Geometry: final body of the model. Coordinates: model frame, mm. A direction names the side the tool comes from. Give positions to 0.01 mm unless a question says otherwise; leave off trailing zeros. Loops run counter-clockwise (first coordinate to the right, second up) from the corner with the lowest first, then second, coordinate; pieces in that order, holes last. Notation, with made-up numbers: (63.25, 43.25) - (86.25, 43.25) arc R19 ccw to (86.25, 66.25) - close; hole circle Ø8 at (-3, 36). An arc over 180 degrees is marked (long way). Use one line per item in the form item = value.
```python
from build123d import *

# Parameters (mm, degrees)
SKETCH1_R    = 5
SPIGOT_DEPTH = 14
BODY_START   = 14
SKETCH2_R    = 7
BODY_DEPTH   = 22
SPOUT_START  = -38
SKETCH3_R    = 5
SPOUT_DEPTH  = 38
LEVER_START  = 6
SKETCH4_W    = 10
SKETCH4_H    = 6
LEVER_DEPTH  = 22


with BuildPart() as part:
    # Sketch1 → Spigot (new body)
    with BuildSketch(Plane.XY):
        Circle(SKETCH1_R)
    extrude(amount=SPIGOT_DEPTH)

    # Sketch2 → Body (add)
    with BuildSketch(Plane.XY.offset(BODY_START)):
        Circle(SKETCH2_R)
    extrude(amount=BODY_DEPTH)

    # Sketch3 → Spout (add)
    with BuildSketch(Plane(origin=(0, 0, 0), x_dir=(1, 0, 0), z_dir=(0, 1, 0)).offset(SPOUT_START)):
        with Locations(Location((0, -30, 0), (0, 0, 90))):
            Circle(SKETCH3_R)
    extrude(amount=SPOUT_DEPTH)

    # Sketch4 → Lever (add)
    with BuildSketch(Plane(origin=(0, 0, 0), x_dir=(1, 0, 0), z_dir=(0, 1, 0)).offset(LEVER_START)):
        with Locations((0, -26)):
            Rectangle(SKETCH4_W, SKETCH4_H)
    extrude(amount=LEVER_DEPTH)


solid = part.part
```
(1) Access query for faces 1 (the face through (-1.5, -21.68, 25.23)), 2 (the face through (-1.08, -4.88, 6.9)), 3 (the face through (-5, 17, 26)), 4 (the face through (5, 17, 26)). Directions: +Z, -Z, +X, -X, +Y, -Y. A direction counts if a zero-diameter tool reaches every point of the face in a straight line with its end or side. Return the directions, or none.
Solution:
face_1 = -Y
face_2 = -Z
face_3 = +Z, -Z, -X, +Y
face_4 = +Z, -Z, +X, +Y
(2) Cut plane B-B (y = 0). Return the cut outline in (x, z).
Solution:
outline = (-7, 14) - (-5, 14) - (-5, 0) - (5, 0) - (5, 14) - (7, 14) - (7, 36) - (-7, 36) - close
(3) Material intervals for L1, parallel to Y at x = 0, z = 19; L2, parallel to Z at x = -1.25, y = 23; L3, parallel to Z at x = 6.25, y = -2.5, sorted ascending. Write a range as from..to.
Solution:
L1 = -7..7
L2 = 23..29
L3 = 14..36
(4) Cut plane D-D (x = 2.75). Return the cut outline in (y, z), plus the area to 3 significant figures.
Solution:
outline = (-38, 25.82) - (-6.44, 25.82) - (-6.44, 14) - (-4.18, 14) - (-4.18, 0) - (4.18, 0) - (4.18, 14) - (6.44, 14) - (6.44, 23) - (28, 23) - (28, 29) - (6.44, 29) - (6.44, 36) - (-6.44, 36) - (-6.44, 34.18) - (-38, 34.18) - close
area = 793 mm2
(5) Cut plane A-A (x = 0). Return the cut outline in (y, z).
Solution:
outline = (-38, 25) - (-7, 25) - (-7, 14) - (-5, 14) - (-5, 0) - (5, 0) - (5, 14) - (7, 14) - (7, 23) - (28, 23) - (28, 29) - (7, 29) - (7, 36) - (-7, 36) - (-7, 35) - (-38, 35) - close
(6) Pin query (flat end, axial travel): P1, Ø1, axis at y = 6.5, z = 7, coming from the -X side; P2, Ø5, axis at y = 17, z = 25.5, coming from the -X side; P3, Ø1.5, axis at x = -4.5, z = 26, coming from the -Y side; P4, Ø3, axis at x = -1.5, y = -25, coming from the +Z side. Return the tip coordinate at first contact, or that it passes through.
Solution:
P1 = through
P2 = -5
P3 = -5.91
P4 = 35
(7) Pull-direction query (Y, two-part tool) for faces 5 (the face through (0, 0, 36)), 6 (the face through (4, 6, 26)), 7 (the face through (0, -38, 30)); classes: released by +Y, released by -Y, zero draft, split by the parting line, or undercut.
Solution:
face_5 = zero draft
face_6 = undercut
face_7 = released by -Y
(8) Cut plane C-C (z = 16). Return the cut outline in (x, y).
Solution:
outline = circle Ø14 at (0, 0)
